Can you work these out from the model? Positions are in its coordinate system, mm. A direction names the side the tool comes from. Coordinates: 2 decimals unless noted, no trailing zeros. Write each loop counter-clockwise with the first axis right and the second up, starting at its lowest first coordinate (ties: lowest second). Pieces come first, ordered by that corner, then holes. Notation, with made-up numbers: M -12.5,16.5 L 32.5,16.5 A8 cw 32.5,21.5 Z; hole C 53,25.5 d3. An arc over 180 degrees is marked long. Use one line per item in the form item = value. Start each with the question number.
```python
from build123d import *

# Parameters (mm, degrees)
SKETCH1_R                                           = 7.14375
BOSS_EXTRUDE1_DEPTH                                 = 4.7625
CBORE_FOR_00_BINDING_HEAD_MACHINE_SCREW_D           = 7.9375
CBORE_FOR_00_BINDING_HEAD_MACHINE_SCREW_CBORE_D     = 11.1125
CBORE_FOR_00_BINDING_HEAD_MACHINE_SCREW_CBORE_DEPTH = 3.175
FILLET2_R                                           = 0.508


with BuildPart() as part:
    # Sketch1 → Boss-Extrude1 (new body)
    with BuildSketch(Plane(origin=(0, 0, 0), x_dir=(1, 0, 0), z_dir=(0, 1, 0))):
        with Locations(Location((0, 0, 0), (0, 0, 90))):
            Circle(SKETCH1_R)
    extrude(amount=BOSS_EXTRUDE1_DEPTH)

    # CBORE for _00 Binding Head Machine Screw (through all)
    with Locations(Plane(origin=(0, 4.7625, 0), x_dir=(1, 0, 0), z_dir=(0, 1, 0))):
        with Locations((0, 0)):
            CounterBoreHole(CBORE_FOR_00_BINDING_HEAD_MACHINE_SCREW_D / 2, CBORE_FOR_00_BINDING_HEAD_MACHINE_SCREW_CBORE_D / 2, CBORE_FOR_00_BINDING_HEAD_MACHINE_SCREW_CBORE_DEPTH)

    # Fillet2
    fillet2_edges = [part.edges().sort_by_distance(p)[0] for p in [
        (0, 4.7625, 7.14375),
        (-5.55625, 4.7625, 0),
    ]]
    fillet(fillet2_edges, radius=FILLET2_R)


solid = part.part
```
1) Suppose I cut it at A-A on z = 0. Please give me the cut outline in (x, y), and give its area (3 significant figures).
2) Please list where these lines run through material, in increasing order: line 1 (Y direction, x = -4, z = 3); line 2 (X direction, y = 2.5, z = 3.5); line 3 (X direction, y = 2.4, z = 0).
3) Suppose I cut it at C-C on y = 2.5. Please give me the cut outline in (x, z), and give its area (3 significant figures).
4) Will these pins go through, and if not, where does the flat tip stop? pin 1 Ø5 at (x, z) = (0, 0) entering from -Y; pin 2 Ø1 at (y, z) = (1, 2) entering from +X; pin 3 Ø2 at (x, z) = (2, -3.5) entering from +Y.
5) If we mould it in two halves opening along Z, with no side actions, what happens to faces 3 (the face through (-4, 1.588, -1)), 4 (the face through (-0.314, 2.097, 7.137)), 5 (the face through (3, 0, -3))? For each: +Z half, -Z half, draft (parallel to the pull), parting line (faces both ways), or undercut.
6) Which directions (+Z, -Z, +X, -X, +Y, -Y) give clear straight access to the entire face, cutting with the end or side of a thin tool? Please do faces 1 (the face through (0.86, 0.783, 3.874)), 2 (the face through (5.3, 2.94, -1.67)).
7) Suppose I cut it at B-B on x = 0. Please give me the cut outline in (y, z).
Computed values:
q1.outline = M -7.14,0 L -3.97,0 L -3.97,1.59 L -5.56,1.59 L -5.56,4.25 A0.51 ccw -6.06,4.76 L -6.64,4.76 A0.51 ccw -7.14,4.25 Z; M 3.97,0 L 7.14,0 L 7.14,4.25 A0.51 ccw 6.64,4.76 L 6.06,4.76 A0.51 ccw 5.56,4.25 L 5.56,1.59 L 3.97,1.59 Z
q1.area = 19.9 mm²
q2.line_1 = 0 to 1.59
q2.line_2 = -6.23 to -4.32, 4.32 to 6.23
q2.line_3 = -7.14 to -5.56, 5.56 to 7.14
q3.outline = C 0,0 d14.29; hole C 0,0 d11.11
q3.area = 63.3 mm²
q4.pin_1 = through
q4.pin_2 = 6.98
q4.pin_3 = 1.59
q5.face_3 = undercut
q5.face_4 = parting line
q5.face_5 = draft
q6.face_1 = +Y, -Y
q6.face_2 = +Y
q7.outline = M 0,-7.14 L 4.25,-7.14 A0.51 ccw 4.76,-6.64 L 4.76,-6.06 A0.51 ccw 4.25,-5.56 L 1.59,-5.56 L 1.59,-3.97 L 0,-3.97 Z; M 0,3.97 L 1.59,3.97 L 1.59,5.56 L 4.25,5.56 A0.51 ccw 4.76,6.06 L 4.76,6.64 A0.51 ccw 4.25,7.14 L 0,7.14 Z
